Source: three-view drawing plus pictorial views. Frame: mm from the lowest corner of the part. A direction names the side the tool comes from. Give positions to 0.01 mm unless a question says otherwise; leave off trailing zeros. Loops run counter-clockwise (first coordinate to the right, second up) from the corner with the lowest first, then second, coordinate; pieces in that order, holes last.
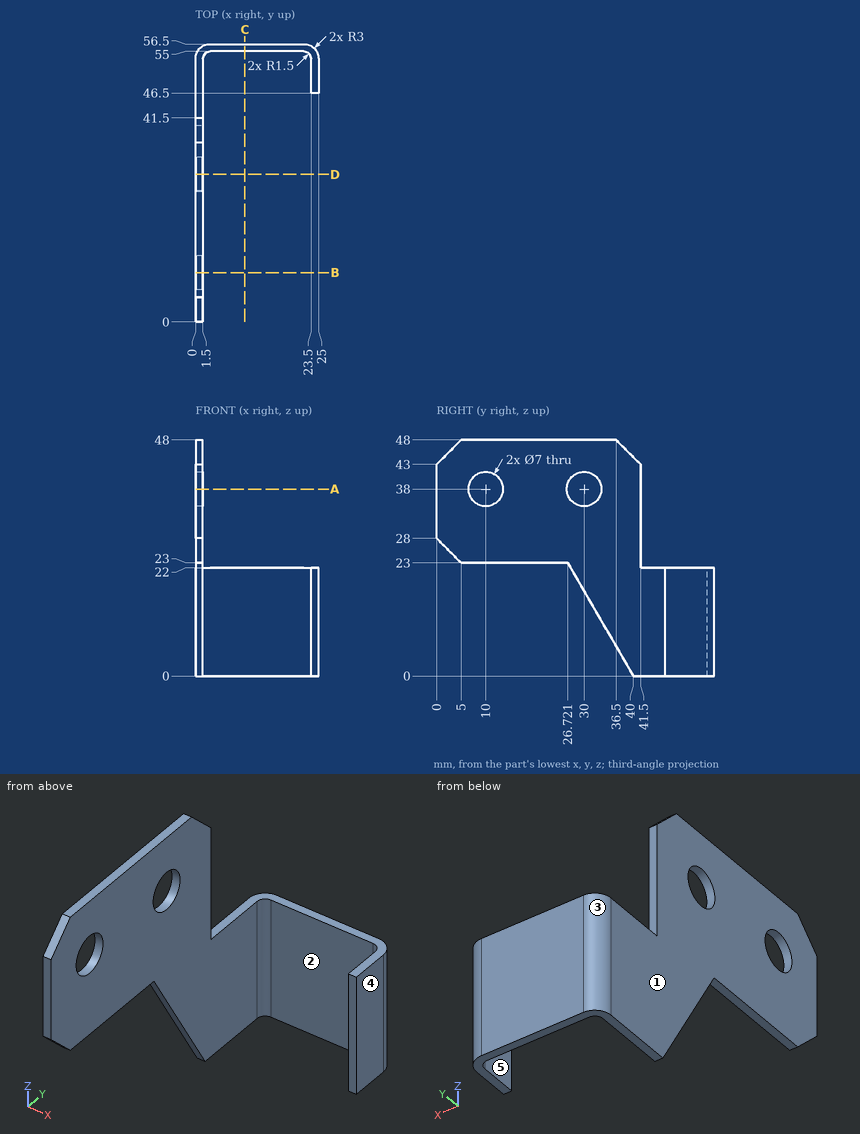
(1) Mould query, pull axis X, two halves, no side actions, for the marked faces 3, 4 and 5. Classes: +X half, -X half, draft (parallel to the pull), parting line (faces both ways), or undercut.
Values follow:
face 3: -X half
face 4: +X half
face 5: undercut
(2) Pin query (flat end, axial travel): pin 1 Ø6.5 at (y, z) = (30, 38) entering from +X; pin 2 Ø10 at (y, z) = (39.5, 16) entering from +X; pin 3 Ø1 at (x, z) = (3, 10.5) entering from -Y; pin 4 Ø1.2 at (x, y) = (0.5, 13.5) entering from -Z. Return the tip coordinate at first contact, or that it passes through.
Values follow:
pin 1: passes through
pin 2: stops at x = 1.5
pin 3: stops at y = 54.91
pin 4: stops at z = 23
(3) Cut plane D-D (y = 30). Return the cut outline in (x, z).
Values follow:
outline: (0, 17.32) - (1.5, 17.32) - (1.5, 34.5) - (0, 34.5) - close; (0, 41.5) - (1.5, 41.5) - (1.5, 48) - (0, 48) - close
(4) Cut plane A-A (z = 38). Return the cut outline in (x, y).
Values follow:
outline: (0, 0) - (1.5, 0) - (1.5, 6.5) - (0, 6.5) - close; (0, 13.5) - (1.5, 13.5) - (1.5, 26.5) - (0, 26.5) - close; (0, 33.5) - (1.5, 33.5) - (1.5, 41.5) - (0, 41.5) - close
(5) Cut plane C-C (x = 10). Return the cut outline in (y, z), and give its area (3 significant figures).
Values follow:
outline: (55, 0) - (56.5, 0) - (56.5, 22) - (55, 22) - close
area: 33.0 mm2
(6) Ray query, probe 1 along Y at (x, z) = (0.9, 38); probe 2 along Y at (x, z) = (13.75, 12.5); probe 3 along X at (y, z) = (7.5, 28). Return the intervals inside material, ascending.
Values follow:
probe 1: y = 0 to 6.5, 13.5 to 26.5, 33.5 to 41.5
probe 2: y = 55 to 56.5
probe 3: x = 0 to 1.5
(7) Reachability of the marked faces 1 and 2 from +Z, -Z, +X, -X, +Y, -Y: full face, straight path, thin tool, end or side. Return the list, or none.
Values follow:
face 1: +Z, -Z, -X, +Y, -Y
face 2: +Z, -Z, -Y
(8) Cut plane B-B (y = 10). Return the cut outline in (x, z).
Values follow:
outline: (0, 23) - (1.5, 23) - (1.5, 34.5) - (0, 34.5) - close; (0, 41.5) - (1.5, 41.5) - (1.5, 48) - (0, 48) - close
